Geometry: final body of the model. Coordinates: model frame, mm. A direction names the side the tool comes from. Give positions to 0.01 mm unless a question says otherwise; leave off trailing zeros. Write each loop counter-clockwise with the first axis right and the second up, starting at its lowest first coordinate (ties: lowest second). Pieces come first, ordered by that corner, then holes. Notation, with made-up numbers: M -13.75,-14 L 24.25,-14 A27 cw 24.25,24 Z; hole C -13,-11 d4. An arc over 180 degrees is marked long. Use a Markdown table: item, result. Add a question column.
(1) Reachability of faces 5 (the flat face through (33, 0, 1156)), 6 (the flat face through (0, -33, 1156)), 7 (the flat face through (3, 58, 21)) from +Z, -Z, +X, -X, +Y, -Y: full face, straight path, thin tool, end or side. Return the list, or none.
(2) Cut plane A-A (z = 1754.5). Output: boundary loops of the cut face in (x, y), plus the area to 3 significant figures.
(3) Material intervals for L1, parallel to Z at x = 0, y = -5.5; L2, parallel to X at y = -5, z = 202.5; L3, parallel to X at y = -4, z = 2444, sorted ascending.
(4) Cut plane B-B (y = 79). Output: boundary loops of the cut face in (x, z), plus the area to 3 significant figures.
(5) Pin query (flat end, axial travel): pin 1 Ø2 at (x, y) = (81.5, 1.5) entering from +Z; pin 2 Ø20 at (y, z) = (15, 976.5) entering from +X; pin 3 Ø10 at (x, z) = (9, 2201) entering from +Y. Return the tip coordinate at first contact, or that it passes through.
(6) Draft query along Y for faces 1 (the flat face through (0, 33, 1156)), 2 (the flat face through (37.5, -1, 1156)), 3 (the flat face through (58, -3, 21)), 4 (the flat face through (-33, 0, 1156)). Return one class per face: released by +Y, released by -Y, zero draft, split by the parting line, or undercut.
```python
from build123d import *

# Parameters (mm, degrees)
F0_W     = 75
F0_H     = 75
F0_W_2   = 66
F0_H_2   = 66
F1_DEPTH = 2344
F2_R     = 30
F3_DEPTH = 9.5
F5_DEPTH = 3
F7_DEPTH = 3


with BuildPart() as f1:
    # F0 (on Top) → F1 (new body)
    with BuildSketch(Plane.XY):
        Rectangle(F0_W, F0_H)
        Rectangle(F0_W_2, F0_H_2, mode=Mode.SUBTRACT)
    extrude(amount=F1_DEPTH)

    # F2 (on Front) → F3 (join, symmetric)
    with BuildSketch(Plane.XZ):
        with BuildLine():
            Line((-50, 2444), (-50, 2294))
            Line((-50, 2294), (50, 2294))
            Line((50, 2294), (50, 2444))
            ThreePointArc((50, 2444), (0, 2494), (-50, 2444))
        make_face()
        with Locations((0, 2444)):
            Circle(F2_R, mode=Mode.SUBTRACT)
    extrude(amount=F3_DEPTH, both=True)

    # F4 (on Front) → F5 (join, symmetric)
    with BuildSketch(Plane.XZ):
        Polygon((37.5, 75), (37.5, 0), (112.5, 0), align=None)
    extrude(amount=F5_DEPTH, both=True)

    # F6 (on Right) → F7 (join, symmetric)
    with BuildSketch(Plane.YZ):
        Polygon((37.5, 75), (37.5, 0), (112.5, 0), align=None)
    extrude(amount=F7_DEPTH, both=True)


solid = f1.part
```
Answer list:
| question | item | result |
|---|---|---|
| 1 | face 5 | -Z |
| 1 | face 6 | +Z, -Z |
| 1 | face 7 | +Z, -Z, +X, +Y |
| 2 | outline | M -37.5,-37.5 L 37.5,-37.5 L 37.5,37.5 L -37.5,37.5 Z; hole M -33,-33 L 33,-33 L 33,33 L -33,33 Z |
| 2 | area | 1,270 mm² |
| 3 | L1 | 2294 to 2414, 2474 to 2494 |
| 3 | L2 | -37.5 to -33, 33 to 37.5 |
| 3 | L3 | -50 to -30, 30 to 50 |
| 4 | outline | M -3,0 L 3,0 L 3,33.5 L -3,33.5 Z |
| 4 | area | 201 mm² |
| 5 | pin 1 | z = 32 |
| 5 | pin 2 | x = 37.5 |
| 5 | pin 3 | y = 37.5 |
| 6 | face 1 | undercut |
| 6 | face 2 | zero draft |
| 6 | face 3 | released by -Y |
| 6 | face 4 | undercut |
